The listing builds one solid part. Answer for the finished solid, in the listing's coordinates (mm). A direction names the side the tool comes from. Round coordinates to 2 decimals unless told otherwise and drop trailing zeros. Write each loop counter-clockwise with the first axis right and the second up, starting at its lowest first coordinate (ties: lowest second). Pieces come first, ordered by that corner, then holes.
from build123d import *

# Parameters (mm, degrees)
F0_R      = 107.5
F1_DEPTH  = 23
F2_R      = 50
F3_DEPTH  = 80
F4_R      = 87.5
F4_R_2    = 50
F5_DEPTH  = 22
F6_R      = 42.5
F6_R_2    = 32.5
F7_DEPTH  = 6
F7_FACE_R = 32.5
F8_DEPTH  = 125.001
F9_R      = 77
F10_DEPTH = 6
F11_R     = 6.5
F12_DEPTH = 25
F13_R     = 8.75
F14_DEPTH = 25


with BuildPart() as f1:
    # F0 (on Top) → F1 (new body)
    with BuildSketch(Plane.XY):
        Circle(F0_R)
    extrude(amount=F1_DEPTH)

    # F2 (on face) → F3 (join)
    with BuildSketch(Plane.XY.offset(23)):
        Circle(F2_R)
    extrude(amount=F3_DEPTH)

    # F4 (on face) → F5 (join)
    with BuildSketch(Plane.XY.offset(103)):
        Circle(F4_R)
        Circle(F4_R_2, mode=Mode.SUBTRACT)
        Circle(F4_R_2)
    extrude(amount=F5_DEPTH)

    # F6 (on face) → F7 (join)
    with BuildSketch(Plane.XY.offset(125)):
        Circle(F6_R)
        Circle(F6_R_2, mode=Mode.SUBTRACT)
    extrude(amount=F7_DEPTH)

    # F7_face (on face) → F8 (cut, through all)
    with BuildSketch(Plane.XY.offset(125)):
        Circle(F7_FACE_R)
    extrude(amount=-F8_DEPTH, mode=Mode.SUBTRACT)

    # F9 (on face) → F10 (cut)
    with BuildSketch(Plane(origin=(0, 0, 0), x_dir=(1, 0, 0), z_dir=(0, 0, -1))):
        Circle(F9_R)
    extrude(amount=-F10_DEPTH, mode=Mode.SUBTRACT)

    # F11 (on face) → F12 (cut)
    with BuildSketch(Plane.XY.offset(125)):
        with Locations((-38.5, 66.683956)):
            Circle(F11_R)
        with Locations((38.5, 66.683956)):
            Circle(F11_R)
        with Locations((71.138724, 29.466624)):
            Circle(F11_R)
        with Locations((71.138724, -29.466624)):
            Circle(F11_R)
        with Locations((29.466624, -71.138724)):
            Circle(F11_R)
        with Locations((-29.466624, -71.138724)):
            Circle(F11_R)
        with Locations((-71.138724, -29.466624)):
            Circle(F11_R)
        with Locations((-71.138724, 29.466624)):
            Circle(F11_R)
    extrude(amount=-F12_DEPTH, mode=Mode.SUBTRACT)

    # F13 (on face) → F14 (cut)
    with BuildSketch(Plane(origin=(0, 0, 0), x_dir=(1, 0, 0), z_dir=(0, 0, -1))):
        with Locations((-62.932504, 62.932504)):
            Circle(F13_R)
        with Locations((62.932504, 62.932504)):
            Circle(F13_R)
        with Locations((89, 0)):
            Circle(F13_R)
        with Locations((44.5, -77.076261)):
            Circle(F13_R)
        with Locations((-44.5, -77.076261)):
            Circle(F13_R)
        with Locations((-89, 0)):
            Circle(F13_R)
    extrude(amount=-F14_DEPTH, mode=Mode.SUBTRACT)


solid = f1.part
1. Section D-D on z = 97.5 is taken. Determine the outline of the cut face in (x, y).
Geometry says:
outline: circle Ø100 at (0, 0); hole circle Ø65 at (0, 0)
2. For a pull along X with two mould halves and no side action, classify faces 1 (the face through (28.62, -64.694, 114.154)), 2 (the face through (-1, -79, 0)), 3 (the face through (-33.727, -25.861, 127.958)) as released by +X, released by -X, zero draft, split by the parting line, or undercut.
Geometry says:
face 1: undercut
face 2: zero draft
face 3: split by the parting line
3. Section C-C on x = -39 is taken. Determine the outline of the cut face in (y, z), plus the area to 3 significant figures.
Geometry says:
outline: (-100.18, 0) - (-66.39, 0) - (-66.39, 6) - (66.39, 6) - (66.39, 0) - (70.27, 0) - (70.27, 23) - (31.29, 23) - (31.29, 103) - (60.2, 103) - (60.2, 125) - (16.89, 125) - (16.89, 131) - (-16.89, 131) - (-16.89, 125) - (-78.33, 125) - (-78.33, 103) - (-31.29, 103) - (-31.29, 23) - (-100.18, 23) - close; (73.16, 103) - (78.33, 103) - (78.33, 125) - (73.16, 125) - close; (83.88, 0) - (100.18, 0) - (100.18, 23) - (83.88, 23) - close
area: 11,900 mm2
4. Given pin 1 (10 mm diameter, centred on x = -75, y = 27, fed in from +Z); pin 2 (12 mm diameter, centred on y = 8.5, z = 88.5, fed in from -X); pin 3 (1.5 mm diameter, centred on y = 13, z = 78, fed in from -X); pin 4 (10.5 mm diameter, centred on x = 71.14, y = -29.47, fed in from -Z), each flat-ended and moving along its own axis, determine where each tip first touches the part or whether it passes through.
Geometry says:
pin 1: stops at z = 125
pin 2: stops at x = -49.94
pin 3: stops at x = -48.48
pin 4: stops at z = 0
5. Section B-B on y = 0 is taken. Give the number of separate pieces and of enclosed holes in the cut face, plus the area to 3 significant figures.
Geometry says:
separate pieces: 4
enclosed holes: 0
area: 7,450 mm2
6. Section A-A on x = 0 is taken. Determine the outline of the cut face in (y, z).
Geometry says:
outline: (-107.5, 0) - (-77, 0) - (-77, 6) - (-32.5, 6) - (-32.5, 131) - (-42.5, 131) - (-42.5, 125) - (-87.5, 125) - (-87.5, 103) - (-50, 103) - (-50, 23) - (-107.5, 23) - close; (32.5, 6) - (77, 6) - (77, 0) - (107.5, 0) - (107.5, 23) - (50, 23) - (50, 103) - (87.5, 103) - (87.5, 125) - (42.5, 125) - (42.5, 131) - (32.5, 131) - close
7. A tool of negligible diameter and unlimited length cuts with its end or side. For faces 4 (the face through (97.346, -2.628, 11.339)), 5 (the face through (65.98, -33.42, 114.15)), 6 (the face through (22, -46, 23)), from which of +Z, -Z, +X, -X, +Y, -Y can it reach the whole face along a straight path? Write none if from no direction.
Geometry says:
face 4: -Z
face 5: +Z
face 6: none
8. Straight lines are drawn through the part: line 1 along Z through (x, y) = (2, 78.5); line 2 along Z through (x, y) = (51.5, 47.5); line 3 along X through (y, z) = (71, 14). For each, find the intervals that lie inside material, in ascending order.
Geometry says:
line 1: z = 0 to 23, 103 to 125
line 2: z = 6 to 23, 103 to 125
line 3: x = -80.72 to -50.8, -38.2 to 38.2, 50.8 to 80.72
